Can you work these out from the drawing? Everything is in mm from the part's minimum corner. Give positions to 0.01 mm unless a question says otherwise; leave off trailing zeros. Write each loop counter-clockwise with the first axis right and the second up, starting at its lowest first coordinate (ties: lowest second). Pieces come first, ordered by that corner, then holes. Notation, with made-up numbers: (84.25, 10) -> (101.25, 10) arc R15 cw to (101.25, 32) -> close; hole circle Ø5 at (65.25, -36.5). An arc over 180 degrees is marked (long way). Return JSON: item names as keys, results as strings.
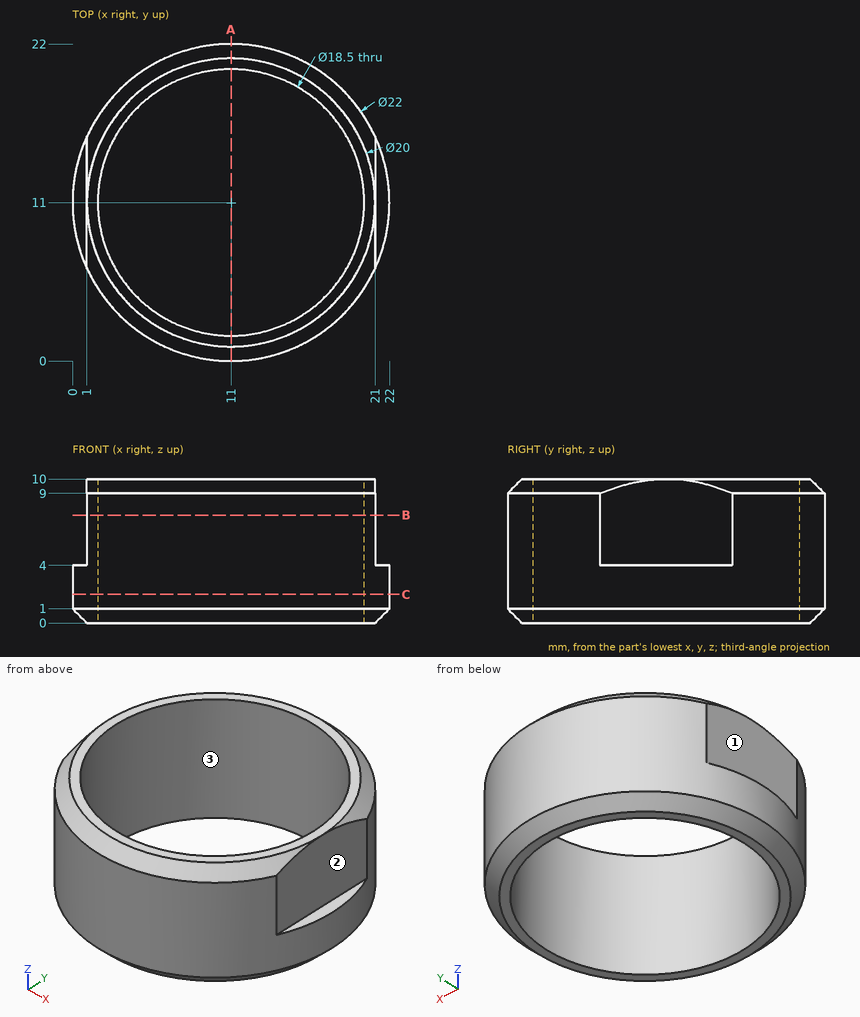
1. Suppose I cut it at B-B, the plane z = 7.5. List the corners of the cut face in (x, y) for me, and give its area (3 significant figures).
Taken from the geometry:
{"outline": "(1, 6.42) arc R11 ccw to (21, 6.42) -> (21, 15.58) arc R11 ccw to (1, 15.58) -> close; hole circle Ø18.5 at (11, 11)", "area": "99.0 mm²"}
2. For pin 1 Ø0.5 at (x, y) = (21.5, 13) entering from +Z; pin 2 Ø6 at (y, z) = (5, 3) entering from +X; pin 3 Ø2 at (y, z) = (12.5, 1) entering from -X, each with a flat end and sliding along its axis, tell me the tip position at first contact or that it passes through.
Taken from the geometry:
{"pin 1": "stops at z = 4", "pin 2": "stops at x = 21.58", "pin 3": "stops at x = 0.01"}
3. Suppose I cut it at A-A, the plane x = 11. List the corners of the cut face in (y, z) for me.
Taken from the geometry:
{"outline": "(0, 1) -> (1, 0) -> (1.75, 0) -> (1.75, 10) -> (1, 10) -> (0, 9) -> close; (20.25, 0) -> (21, 0) -> (22, 1) -> (22, 9) -> (21, 10) -> (20.25, 10) -> close"}
4. If we mould it in two halves opening along X, with no side actions, what happens to the marked faces 1, 2 and 3? For each: released by +X, released by -X, zero draft, split by the parting line, or undercut.
Taken from the geometry:
{"face 1": "released by -X", "face 2": "released by +X", "face 3": "undercut"}
5. Suppose I cut it at C-C, the plane z = 2. List the corners of the cut face in (x, y) for me, and give its area (3 significant figures).
Taken from the geometry:
{"outline": "circle Ø22 at (11, 11); hole circle Ø18.5 at (11, 11)", "area": "111 mm²"}
6. If I drill on line 1 (Y direction, x = 11, z = 2.75); line 2 (Y direction, x = 6.25, z = 7.5); line 3 (X direction, y = 16.25, z = 3), over which ranges is the centre line in solid material (lowest first)? Write a range as [from, to].
Taken from the geometry:
{"line 1": "y = [0, 1.75], [20.25, 22]", "line 2": "y = [1.08, 3.06], [18.94, 20.92]", "line 3": "x = [1.33, 3.38], [18.62, 20.67]"}
